For this review, take the finished solid that the model builds, in its own axes (mm). Face numbers are marked on the shaded views. A direction names the side the tool comes from. Give positions to 0.01 mm unless a question says otherwise; leave off trailing zeros. Order: outer loops, then holes, each group sorted by start corner. A loop starts at its lowest first (then second) coordinate and runs counter-clockwise, first axis right, second up. Notation, with made-up numbers: (0, 36) -> (28, 36) arc R19 ccw to (28, 56) -> close; hole circle Ø4 at (-35.5, -17.5). An arc over 180 degrees is marked (long way). Return JSON: item names as keys, results as strings. Group by question number.
1) To check wall thickness, follow line 1 along Y through (x, z) = (1.75, 49.5); line 2 along X through (y, z) = (-18.5, 22); line 3 along Y through (x, z) = (13.8, 50). State the ranges of each line that lie inside material, in increasing order.
2) Add section B-B (z = 50). Give the boundary of the cut face in (x, y).
3) Add section D-D (y = -44). Give the boundary of the cut face in (x, z).
4) The part is to be moulded in two halves that separate along Y. For the marked faces 3, 4 and 5, say which applies: released by +Y, released by -Y, zero draft, split by the parting line, or undercut.
5) Add section C-C (x = -3.5). Give the boundary of the cut face in (y, z), then the cut area to 3 significant figures.
6) For the marked faces 1 and 2, list the 3-axis set-ups (+Z, -Z, +X, -X, +Y, -Y) from which the entire face can be reached by the end or side of a thin tool; tool diameter is ignored.
7) Add section A-A (y = 40). Give the boundary of the cut face in (x, z), then the cut area to 3 significant figures.
8) Insertion check: P1, Ø4, axis at y = 0.5, z = 39.5, coming from the +X side. The pin has a flat end and moves straight along its axis. Give the tip position at first contact, or say it passes through.
Autodesk Inventor part; units mm, degrees
ref_plane "YZ Plane" through (0, 0, 0) normal (1, 0, 0) x (0, 1, 0)
ref_plane "XZ Plane" through (0, 0, 0) normal (0, 1, 0) x (-1, 0, 0)
ref_plane "XY Plane" through (0, 0, 0) normal (0, 0, 1) x (1, 0, 0)
sketch "Sketch1" plane through (0, 0, 0) normal (0, 0, 1) x (1, 0, 0)
  line L0 (-15, -50) -> (15, -50)
  line L1 (15, -50) -> (15, 50)
  line L2 (15, 50) -> (-15, 50)
  line L3 (-15, 50) -> (-15, -50)
  line L4 (-15, -50) -> (15, 50) construction
  line L5 (15, -50) -> (-15, 50) construction
  line L6 (-13, 48) -> (13, 48)
  line L7 (13, 48) -> (13, -48)
  line L8 (13, -48) -> (-13, -48)
  line L9 (-13, -48) -> (-13, 48)
  point P0 (0, 0)
  dimension "d0" = 30
  dimension "d1" = 100
  dimension "d2" = 2
extrude "Extrusion1" add sketch "Sketch1" along normal blind 60
sketch "Sketch2" plane through (15, -50, 0) normal (1, 0, 0) x (0, 0, -1)
  circle A0 centre (-30, 50) radius 9.65
  line L0 (-30, 100) -> (-30, 50) construction
  line L1 (0, 0) -> (0, 100)
  line L2 (0, 100) -> (-60, 100)
  line L3 (-30, 50) -> (0, 50) construction
  circle A1 centre (-50, 90) radius 2.75
  circle A2 centre (-10, 90) radius 2.75
  circle A3 centre (-20, 10) radius 2.75
  circle A4 centre (-50, 10) radius 2.75
  line L4 (0, 0) -> (-60, 0)
  dimension "d5" = 19.3
  dimension "d11" = 50
  dimension "d12" = 30
  dimension "d13" = 5.5
  dimension "d14" = 5.5
  dimension "d15" = 5.5
  dimension "d16" = 5.5
  dimension "d18" = 40
  dimension "d19" = 20
  dimension "d20" = 40
  dimension "d21" = 10
  dimension "d22" = 80
  dimension "d23" = 80
  dimension "d24" = 30
  dimension "d25" = 40
extrude "Extrusion2" cut sketch "Sketch2" against normal blind 38.5
sketch "Sketch3" plane through (-13, -48, 0) normal (1, 0, 0) x (0, 0, -1)
  circle A0 centre (-30, 48) radius 9.65
  circle A1 centre (-30, 48) radius 15
  point P0 (0, 48)
  dimension "d8" = 30
extrude "Extrusion3" cut sketch "Sketch3" against normal blind 2 contours A0 | A1
properties part number "transmition Axle Support"
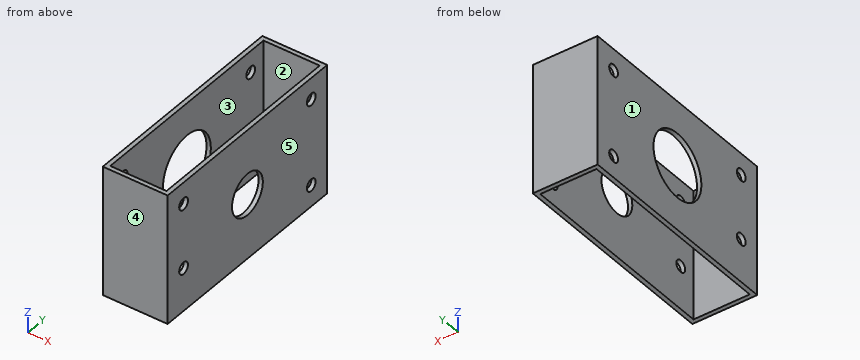
Evaluation:
{
 "1": {"line 1": "-50 to -48, 48 to 50", "line 2": "-15 to -13, 13 to 15", "line 3": "-50 to -42.75, -37.25 to 37.25, 42.75 to 50"},
 "2": {"outline": "(-15, -50) -> (15, -50) -> (15, -42.75) -> (13, -42.75) -> (13, -48) -> (-13, -48) -> (-13, -42.75) -> (-15, -42.75) -> close; (-15, -37.25) -> (-13, -37.25) -> (-13, 37.25) -> (-15, 37.25) -> close; (-15, 42.75) -> (-13, 42.75) -> (-13, 48) -> (13, 48) -> (13, 42.75) -> (15, 42.75) -> (15, 50) -> (-15, 50) -> close; (13, -37.25) -> (15, -37.25) -> (15, 37.25) -> (13, 37.25) -> close"},
 "3": {"outline": "(-15, 0) -> (-13, 0) -> (-13, 60) -> (-15, 60) -> close; (13, 0) -> (15, 0) -> (15, 60) -> (13, 60) -> close"},
 "4": {"face 3": "undercut", "face 4": "released by -Y", "face 5": "zero draft"},
 "5": {"outline": "(-50, 0) -> (-48, 0) -> (-48, 60) -> (-50, 60) -> close; (48, 0) -> (50, 0) -> (50, 60) -> (48, 60) -> close", "area": "240 mm^2"},
 "6": {"face 1": "+Z, -Z, -X, +Y, -Y", "face 2": "+Z, -Z"},
 "7": {"outline": "(-15, 0) -> (-13, 0) -> (-13, 7.25) -> (-15, 7.25) -> close; (-15, 12.75) -> (-13, 12.75) -> (-13, 47.25) -> (-15, 47.25) -> close; (-15, 52.75) -> (-13, 52.75) -> (-13, 60) -> (-15, 60) -> close; (13, 0) -> (15, 0) -> (15, 7.25) -> (13, 7.25) -> close; (13, 12.75) -> (15, 12.75) -> (15, 47.25) -> (13, 47.25) -> close; (13, 52.75) -> (15, 52.75) -> (15, 60) -> (13, 60) -> close", "area": "196 mm^2"},
 "8": {"P1": "x = 15"}
}
